Study the drawing (mm; zero at the part's minimum x, y, z) and answer. Coordinates: 2 decimals unless noted, no trailing zeros. Order: outer loops, then holes, each group sorted by start corner. A loop starts at its lowest first (then second) coordinate and runs counter-clockwise, first axis right, second up. Notation, with made-up numbers: (12.25, -30) -> (30.25, -30) arc R36 cw to (30.25, 9) -> close; hole circle Ø8 at (9.5, 59.25). An arc over 180 degrees is marked (long way). Answer as CSV lines item,"result". Start each with the question number.
Item 1: This flat-tipped pin is pushed along its axis until it touches: pin 1 Ø5 at (x, z) = (15.26, 2.54) entering from -Y. Where does it stop, or does it pass through?
Item 2: Section B-B (y = 1.1) is taken. Count the separate pieces of the cut face and the enclosed holes in it, then the cut area to 3 significant figures.
Item 3: Straight lines are drawn through the part: L1, parallel to X at y = 0.3, z = 22.86; L2, parallel to X at y = 1.1, z = 16.51; L3, parallel to Z at x = 14, y = 0.3. For each, find the intervals that lie inside material, in ascending order.
Item 4: Section A-A (z = 8.75) is taken. Write down the section's boundary in (x, y).
Item 5: Section C-C (z = 11.43) is taken. Write down the section's boundary in (x, y).
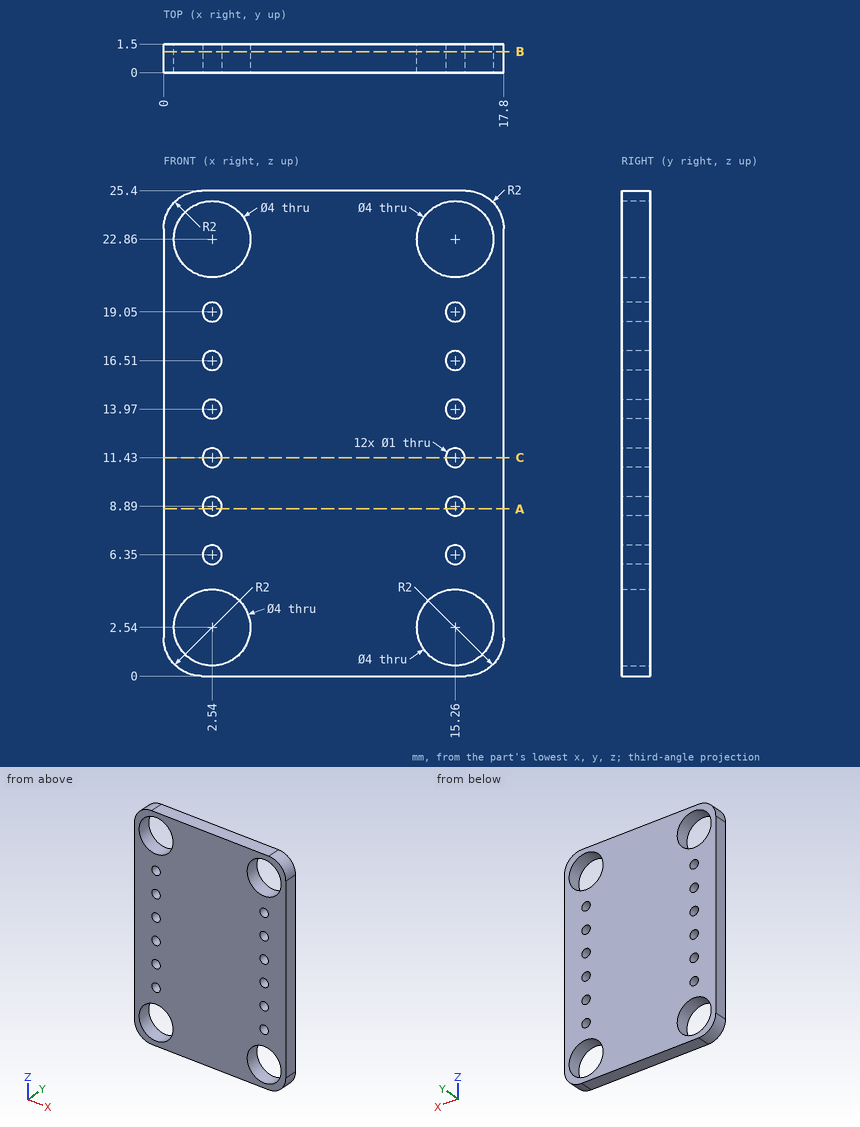
Checked values:
1,pin 1,"stops at y = 0"
2,separate pieces,"1"
2,enclosed holes,"16"
2,area,"389 mm^2"
3,L1,"x = 0 to 0.54, 4.54 to 13.26, 17.26 to 17.8"
3,L2,"x = 0 to 2.04, 3.04 to 14.76, 15.76 to 17.8"
3,L3,"z = 0 to 0.99, 4.09 to 21.31, 24.41 to 25.4"
4,outline,"(0, 0) -> (2.06, 0) -> (2.06, 1.5) -> (0, 1.5) -> close; (3.02, 0) -> (14.78, 0) -> (14.78, 1.5) -> (3.02, 1.5) -> close; (15.74, 0) -> (17.8, 0) -> (17.8, 1.5) -> (15.74, 1.5) -> close"
5,outline,"(0, 0) -> (2.04, 0) -> (2.04, 1.5) -> (0, 1.5) -> close; (3.04, 0) -> (14.76, 0) -> (14.76, 1.5) -> (3.04, 1.5) -> close; (15.76, 0) -> (17.8, 0) -> (17.8, 1.5) -> (15.76, 1.5) -> close"
